from build123d import *

# Parameters (mm, degrees)
CROQUIS1_R                             = 7.5
SALIENTE_EXTRUIR1_DEPTH                = 20
CROQUIS2_W                             = 5
CROQUIS2_H                             = 4
SALIENTE_EXTRUIR2_DEPTH                = 4
CROQUIS4_W                             = 8
CROQUIS4_H                             = 4
SALIENTE_EXTRUIR4_DEPTH                = 4
CORTAR_EXTRUIR1_REACH                  = 28.879
CROQUIS6_W                             = 5
CROQUIS6_H                             = 4
CROQUIS6_W_2                           = 2.5
CROQUIS7_R                             = 1
CORTAR_EXTRUIR2_DEPTH                  = 5
CORTAR_EXTRUIR3_REACH                  = 28.879
CORTAR_EXTRUIR3_END_RADIUS             = 7.5
CROQUIS8_R                             = 2
CORTAR_EXTRUIR3_DIRECTION_2_REACH      = 28.879
CORTAR_EXTRUIR3_DIRECTION_2_END_RADIUS = 7.5
CROQUIS9_W                             = 4
CROQUIS9_H                             = 4
CORTAR_EXTRUIR4_DEPTH                  = 5


with BuildPart() as part:
    # Croquis1 → Saliente-Extruir1 (new body)
    with BuildSketch(Plane.XY):
        Circle(CROQUIS1_R)
    extrude(amount=SALIENTE_EXTRUIR1_DEPTH)

    # Croquis2 → Saliente-Extruir2 (add)
    with BuildSketch(Plane.XY.offset(20)):
        Rectangle(CROQUIS2_W, CROQUIS2_H)
    extrude(amount=SALIENTE_EXTRUIR2_DEPTH)

    # Croquis4 → Saliente-Extruir4 (add)
    with BuildSketch(Plane(origin=(0, 0, 0), x_dir=(-1, 0, 0), z_dir=(0, 0, -1))):
        Rectangle(CROQUIS4_W, CROQUIS4_H)
    extrude(amount=SALIENTE_EXTRUIR4_DEPTH)

    # Croquis6 → Cortar-Extruir1 (cut, up to next)
    with BuildSketch(Plane(origin=(0, 2, 0), x_dir=(1, 0, 0), z_dir=(0, 1, 0)), mode=Mode.PRIVATE) as cortar_extruir1_sk1:
        with Locations((0, 2)):
            Rectangle(CROQUIS6_W, CROQUIS6_H)
    cortar_extruir1_tool1 = extrude(cortar_extruir1_sk1.sketch, amount=-CORTAR_EXTRUIR1_REACH, mode=Mode.PRIVATE) & part.part
    # Croquis6 → Cortar-Extruir1 (cut, up to next)
    with BuildSketch(Plane(origin=(0, 2, 0), x_dir=(1, 0, 0), z_dir=(0, 1, 0)), mode=Mode.PRIVATE) as cortar_extruir1_sk2:
        with Locations((0, -22)):
            Rectangle(CROQUIS6_W_2, CROQUIS6_H)
    cortar_extruir1_tool2 = extrude(cortar_extruir1_sk2.sketch, amount=-CORTAR_EXTRUIR1_REACH, mode=Mode.PRIVATE) & part.part
    add(cortar_extruir1_tool1.solids().sort_by_distance((0, 2, -2))[0], mode=Mode.SUBTRACT)
    add(cortar_extruir1_tool2.solids().sort_by_distance((0, 2, 22))[0], mode=Mode.SUBTRACT)

    # Croquis7 → Cortar-Extruir2 (cut)
    with BuildSketch(Plane.ZY.offset(4)):
        with Locations((-2.5, 0)):
            Circle(CROQUIS7_R)
        with Locations((22.5, 0)):
            Circle(CROQUIS7_R)
    extrude(amount=-CORTAR_EXTRUIR2_DEPTH, mode=Mode.SUBTRACT)

    # Cortar-Extruir3: up to this cylinder (the profile starts inside it)
    cortar_extruir3_end = Plane(origin=(0, 0, 10), z_dir=(0, 0, -1)) * Cylinder(CORTAR_EXTRUIR3_END_RADIUS, 73.758, mode=Mode.PRIVATE)
    # Croquis8 → Cortar-Extruir3 (cut, up to the surface)
    with BuildSketch(Plane(origin=(0, 2, 0), x_dir=(1, 0, 0), z_dir=(0, 1, 0)), mode=Mode.PRIVATE) as cortar_extruir3_sk1:
        with Locations(Location((0, -10, 0), (0, 0, 90))):
            Circle(CROQUIS8_R)
    cortar_extruir3_tool1 = extrude(cortar_extruir3_sk1.sketch, amount=-CORTAR_EXTRUIR3_REACH, mode=Mode.PRIVATE) & cortar_extruir3_end
    add(cortar_extruir3_tool1.solids().sort_by_distance((0, 2, 10))[0], mode=Mode.SUBTRACT)

    # Cortar-Extruir3 direction 2: up to this cylinder (the profile starts inside it)
    cortar_extruir3_direction_2_end = Plane(origin=(0, 0, 10), z_dir=(0, 0, -1)) * Cylinder(CORTAR_EXTRUIR3_DIRECTION_2_END_RADIUS, 73.758, mode=Mode.PRIVATE)
    # Croquis8 → Cortar-Extruir3 direction 2 (cut, up to the surface)
    with BuildSketch(Plane(origin=(0, 2, 0), x_dir=(1, 0, 0), z_dir=(0, 1, 0)), mode=Mode.PRIVATE) as cortar_extruir3_direction_2_sk1:
        with Locations(Location((0, -10, 0), (0, 0, 90))):
            Circle(CROQUIS8_R)
    cortar_extruir3_direction_2_tool1 = extrude(cortar_extruir3_direction_2_sk1.sketch, amount=CORTAR_EXTRUIR3_DIRECTION_2_REACH, mode=Mode.PRIVATE) & cortar_extruir3_direction_2_end
    add(cortar_extruir3_direction_2_tool1.solids().sort_by_distance((0, 2, 10))[0], mode=Mode.SUBTRACT)

    # Croquis9 → Cortar-Extruir4 (cut)
    with BuildSketch(Plane(origin=(2.5, 0, 0), x_dir=(0, 0, -1), z_dir=(1, 0, 0))):
        with Locations((-22, 0)):
            Rectangle(CROQUIS9_W, CROQUIS9_H)
    extrude(amount=-CORTAR_EXTRUIR4_DEPTH, mode=Mode.SUBTRACT)


solid = part.part
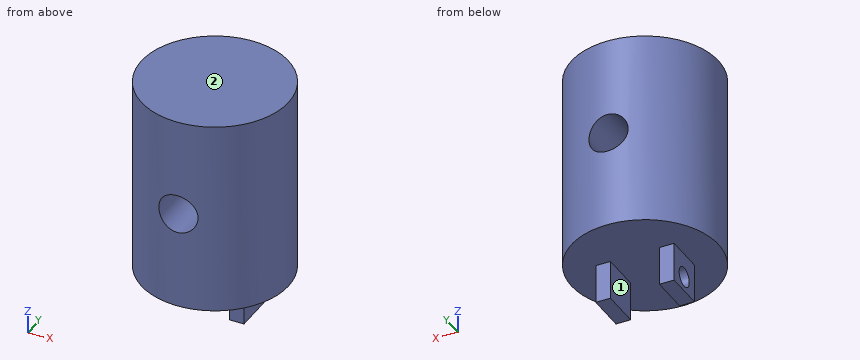
Here's how the part is built. I have some questions about the finished solid (model axes, mm). Face numbers are marked on the shaded views. A direction names the side the tool comes from. Coordinates: 2 decimals unless noted, no trailing zeros. Order: outer loops, then holes, each group sorted by start corner. A loop starts at its lowest first (then second) coordinate and runs counter-clockwise, first axis right, second up. Notation, with made-up numbers: M -5.75,63 L 44.25,63 A34 cw 44.25,100 Z; hole C 42,-24.5 d5. An arc over 180 degrees is marked long. Answer as CSV lines item,"result". Start each with the question number.
1. I want a section at D-D, the plane y = -5. Write out the boundary of the cut face in (x, z), and give its area (3 significant figures).
2. I want a section at A-A, the plane y = 0. Write out the boundary of the cut face in (x, z).
3. I want a section at B-B, the plane z = -2.5. Write out the boundary of the cut face in (x, y), and give its area (3 significant figures).
4. I need wall thicknesses on line 1 (Y direction, x = -3.55, z = -2.5); line 2 (X direction, y = 4.8, z = 10); line 3 (Z direction, x = -2.5, y = -7). Which ranges of each line are inside material? Lowest first, please. Write a range as [from, to].
5. For pin 1 (6.5 mm diameter, centred on x = 0, z = 10, fed in from +Y); pin 2 (4.5 mm diameter, centred on y = -0.5, z = -2.5, fed in from +X); pin 3 (1.5 mm diameter, centred on y = -3, z = 15.5, fed in from -X); pin 4 (3 mm diameter, centred on y = -6, z = 8.5, fed in from -X), each with a flat end and sliding along its axis, tell me the tip position at first contact or that it passes through.
6. I want a section at C-C, the plane x = 1.25. Write out the boundary of the cut face in (y, z), and give its area (3 significant figures).
7. On a 3-axis mill with a long thin cutter (end or side, diameter ignored), from which of +Z, -Z, +X, -X, +Y, -Y can I reach the whole of each face in a straight line? I mean the marked faces 1 and 2. Say none if no direction works.
Recorded:
1,outline,"M -5.59,0 L 5.59,0 L 5.59,20 L -5.59,20 Z; hole C 0,10 d4"
1,area,"211 mm2"
2,outline,"M -7.5,0 L -4,0 L -4,-1.5 L -2.5,-1.5 L -2.5,0 L 2.5,0 L 2.5,-4 L 4,-4 L 4,0 L 7.5,0 L 7.5,20 L -7.5,20 Z; M -4,-4 L -2.5,-4 L -2.5,-3.5 L -4,-3.5 Z; hole C 0,10 d4"
3,outline,"M -4,-2 L -2.5,-2 L -2.5,-1 L -4,-1 Z; M -4,1 L -2.5,1 L -2.5,2 L -4,2 Z; M 2.5,-2 L 4,-2 L 4,2 L 2.5,2 Z"
3,area,"9.00 mm2"
4,line 1,"y = [-2, -1], [1, 2]"
4,line 2,"x = [-5.76, -2], [2, 5.76]"
4,line 3,"z = [0, 20]"
5,pin 1,"stops at y = 7.5"
5,pin 2,"stops at x = 4"
5,pin 3,"stops at x = -7.15"
5,pin 4,"stops at x = -6"
6,outline,"M -7.4,0 L 7.4,0 L 7.4,8.44 L -7.4,8.44 Z; M -7.4,11.56 L 7.4,11.56 L 7.4,20 L -7.4,20 Z"
6,area,"250 mm2"
7,face 1,"-Z, +Y, -Y"
7,face 2,"+Z, +X, -X, +Y, -Y"
